Build history of the part. All positions in model axes, mm. Face numbers are marked on the shaded views. Round coordinates to 2 decimals unless told otherwise and drop trailing zeros. Write each loop counter-clockwise with the first axis right and the second up, starting at its lowest first coordinate (ties: lowest second). Pieces come first, ordered by that corner, then holes.
from build123d import *

# Parameters (mm, degrees)
SKETCH1_R            = 29
SKETCH1_R_2          = 14
SKETCH1_R_3          = 1
BOSS_EXTRUDE1_DEPTH  = 3
SKETCH2_R            = 19
SKETCH2_R_2          = 16
BOSS_EXTRUDE2_DEPTH  = 9
M4_CLEARANCE_HOLE1_D = 4.5
CHAMFER1_SIZE        = 0.5


with BuildPart() as part:
    # Sketch1 → Boss-Extrude1 (new body)
    with BuildSketch(Plane(origin=(0, 0, 0), x_dir=(1, 0, 0), z_dir=(0, 1, 0))):
        with Locations(Location((0, 0, 0), (0, 0, 270))):
            Circle(SKETCH1_R)
        with Locations(Location((0, 0, 0), (0, 0, 270))):
            Circle(SKETCH1_R_2, mode=Mode.SUBTRACT)
        with Locations(Location((0, 24, 0), (0, 0, 270))):
            Circle(SKETCH1_R_3, mode=Mode.SUBTRACT)
        with Locations(Location((24, 0, 0), (0, 0, 270))):
            Circle(SKETCH1_R_3, mode=Mode.SUBTRACT)
        with Locations(Location((0, -24, 0), (0, 0, 270))):
            Circle(SKETCH1_R_3, mode=Mode.SUBTRACT)
        with Locations(Location((-24, 0, 0), (0, 0, 270))):
            Circle(SKETCH1_R_3, mode=Mode.SUBTRACT)
    extrude(amount=BOSS_EXTRUDE1_DEPTH)

    # Sketch2 → Boss-Extrude2 (add)
    with BuildSketch(Plane(origin=(0, 3, 0), x_dir=(1, 0, 0), z_dir=(0, 1, 0))):
        with Locations(Location((0, 0, 0), (0, 0, 270))):
            Circle(SKETCH2_R)
        with Locations(Location((0, 0, 0), (0, 0, 270))):
            Circle(SKETCH2_R_2, mode=Mode.SUBTRACT)
    extrude(amount=BOSS_EXTRUDE2_DEPTH)

    # M4 Clearance Hole1 (through all)
    with Locations(Plane(origin=(0, 3, 0), x_dir=(1, 0, 0), z_dir=(0, 1, 0))):
        with Locations((0, 24), (24, 0), (0, -24), (-24, 0)):
            Hole(M4_CLEARANCE_HOLE1_D / 2)

    # Chamfer1
    chamfer1_edges = [part.edges().sort_by_distance(p)[0] for p in [
        (0, 12, -19),
        (0, 12, -16),
    ]]
    chamfer(chamfer1_edges, length=CHAMFER1_SIZE)


solid = part.part
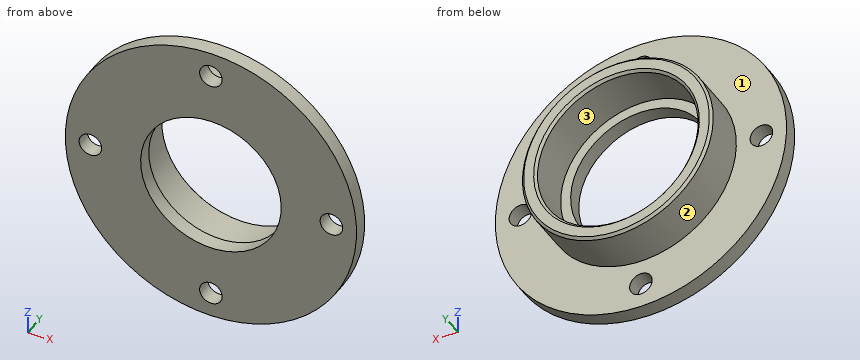
1) Slice it at D-D (x = -24). Write the cut outline in (y, z).
Results:
outline: (0, -16.28) - (3, -16.28) - (3, -2.25) - (0, -2.25) - close; (0, 2.25) - (3, 2.25) - (3, 16.28) - (0, 16.28) - close
2) Mould opens along Z. For the marked faces 1, 2 and 3 say: released by +Z, released by -Z, zero draft, split by the parting line, or undercut.
Results:
face 1: zero draft
face 2: split by the parting line
face 3: undercut
3) Slice it at B-B (z = 0). Write the cut outline in (x, y).
Results:
outline: (-29, 0) - (-26.25, 0) - (-26.25, 3) - (-29, 3) - close; (-21.75, 0) - (-14, 0) - (-14, 3) - (-16, 3) - (-16, 11.5) - (-16.5, 12) - (-18.5, 12) - (-19, 11.5) - (-19, 3) - (-21.75, 3) - close; (14, 0) - (21.75, 0) - (21.75, 3) - (19, 3) - (19, 11.5) - (18.5, 12) - (16.5, 12) - (16, 11.5) - (16, 3) - (14, 3) - close; (26.25, 0) - (29, 0) - (29, 3) - (26.25, 3) - close
4) Pin check, flat tips, straight feed: pin 1 Ø4 at (y, z) = (10.5, -7) entering from -X; pin 2 Ø5 at (x, y) = (-5, 1.5) entering from -Z; pin 3 Ø6 at (x, z) = (0, -24) entering from +Y. Stop position of each tip, or through.
Results:
pin 1: stops at x = -18.33
pin 2: stops at z = -28.89
pin 3: stops at y = 3
5) Wall check: L1, parallel to Z at x = 0.5, y = 8.25; L2, parallel to X at y = 1.75, z = 2; L3, parallel to Y at x = -6.5, z = 22. Give the ranges that are in metal, low to high.
Results:
L1: z = -18.99 to -15.99, 15.99 to 18.99
L2: x = -28.93 to -25.03, -22.97 to -13.86, 13.86 to 22.97, 25.03 to 28.93
L3: y = 0 to 3
6) Slice it at C-C (y = 1.5). Write the cut outline in (x, z).
Results:
outline: circle Ø58 at (0, 0); hole circle Ø4.5 at (-24, 0); hole circle Ø28 at (0, 0); hole circle Ø4.5 at (0, -24); hole circle Ø4.5 at (0, 24); hole circle Ø4.5 at (24, 0)
7) Slice it at A-A (x = 0). Write the cut outline in (y, z).
Results:
outline: (0, -29) - (3, -29) - (3, -26.25) - (0, -26.25) - close; (0, -21.75) - (3, -21.75) - (3, -19) - (11.5, -19) - (12, -18.5) - (12, -16.5) - (11.5, -16) - (3, -16) - (3, -14) - (0, -14) - close; (0, 14) - (3, 14) - (3, 16) - (11.5, 16) - (12, 16.5) - (12, 18.5) - (11.5, 19) - (3, 19) - (3, 21.75) - (0, 21.75) - close; (0, 26.25) - (3, 26.25) - (3, 29) - (0, 29) - close
